Autodesk Inventor part; units mm, degrees
ref_plane "YZ Plane" through (0, 0, 0) normal (1, 0, 0) x (0, 1, 0)
ref_plane "XZ Plane" through (0, 0, 0) normal (0, 1, 0) x (-1, 0, 0)
ref_plane "XY Plane" through (0, 0, 0) normal (0, 0, 1) x (1, 0, 0)
sketch "Sketch1" plane through (0, 0, 0) normal (0, 1, 0) x (-1, 0, 0)
  line L0 (8.5925, 12.671) -> (-4.1075, 12.671)
  line L1 (-4.1075, 12.671) -> (-4.1075, -304.829)
  line L2 (-4.1075, -304.829) -> (8.5925, -304.829)
  line L3 (8.5925, -304.829) -> (8.5925, 12.671)
  point P0 (0, 0)
  dimension "d0" = 12.7
  dimension "d1" = 317.5
extrude "Plate1" add sketch "Sketch1" along normal blind 3.048
fillet "Corner Round1" radius 3.175 4 edges at (4.1075, 1.524, 12.671) (-8.5925, 1.524, 12.671) (-8.5925, 1.524, -304.829) (4.1075, 1.524, -304.829)
sketch "Sketch2" plane through (0, 3.048, 0) normal (0, 1, 0) x (1, 0, 0)
  line L0 (0.9325, -12.671) -> (-5.4175, -12.671)
  line L1 (4.1075, 301.654) -> (4.1075, -9.496)
  line L2 (-5.4175, 304.829) -> (0.9325, 304.829)
  point P0 (0, 0)
  point P1 (-2.2425, -6.321)
  point P2 (-2.2425, 298.479)
  dimension "d4" = 6.35
  dimension "d5" = 6.35
  dimension "d6" = 6.35
  dimension "d7" = 6.35
hole "Hole1" at (-2.2425, 3.048, 6.321) at (-2.2425, 3.048, -298.479) direction (0, -1, 0) diameter 3.2766 end through all
sketch "Sketch3" plane through (0, 3.048, 0) normal (0, 1, 0) x (1, 0, 0)
  line L0 (4.1075, 301.654) -> (4.1075, -9.496)
  circle A0 centre (-2.2425, 298.479) radius 1.6383
  point P0 (0, 0)
  point P1 (-2.2425, 285.779)
  point P2 (-2.2425, 147.6284)
  dimension "d15" = 6.35
  dimension "d16" = 6.35
  dimension "d17" = 138.1506
  dimension "d18" = 12.7
hole "Hole2" at (-2.2425, 3.048, -285.779) at (-2.2425, 3.048, -147.6284) direction (0, -1, 0) diameter 4.9784 end through all
equation "\"BendRadius\" = Thickness"
equation "\"BendReliefWidth\" = Thickness"
equation "\"BendReliefDepth\" = 0.5 * Thickness"
equation "\"CornerReliefSize\" = 4 * Thickness"
equation "\"MinimumRemnant\" = 2 * Thickness"
equation "\"TransitionRadius\" = BendRadius"
equation "\"JacobiRadiusSize\" = BendRadius"
equation "\"GapSize\" = Thickness"
equation "\"d2\" = BendRadius"
properties part number "Compressor_Strut" material "Aluminum 6061"
CAD build for the part. Positions are in the model's coordinates, mm. Coordinates: 2 decimals unless noted, no trailing zeros. Answer as CSV lines item,"result".
1) Flat gauge pin, fed straight in: P1, Ø2, axis at x = -2.24, z = 6.32, coming from the +Y side. Where does the tip first touch, or does it go through?
Verdict:
P1,"through"
2) Mould opens along X. For faces 1 (the cylindrical face through (-2.99, 1.503, -145.254)), 2 (the flat face through (-2, 3.048, -144)) say: released by +X, released by -X, zero draft, split by the parting line, or undercut.
Verdict:
face 1,"undercut"
face 2,"zero draft"
3) Drill centre lines: L1, parallel to Z at x = -2, y = 1.35; L2, parallel to Z at x = -4.5, y = 1.25; L3, parallel to Z at x = -4, y = 2.45. Where is each one in solid material? Low to high. Write a range as from..to.
Verdict:
L1,"-304.83..-300.1, -296.86..-288.26, -283.3..-150.11, -145.15..4.7, 7.94..12.67"
L2,"-304.83..-286.83, -284.73..-148.68, -146.58..12.67"
L3,"-304.83..-287.54, -284.02..-149.39, -145.87..12.67"
4) Cut at A-A (y = 0.6). Give the number of separate pieces and of enclosed holes in the cut face, then the cut area to 3 significant figures.
Verdict:
separate pieces,"1"
enclosed holes,"4"
area,"3,970 mm2"
